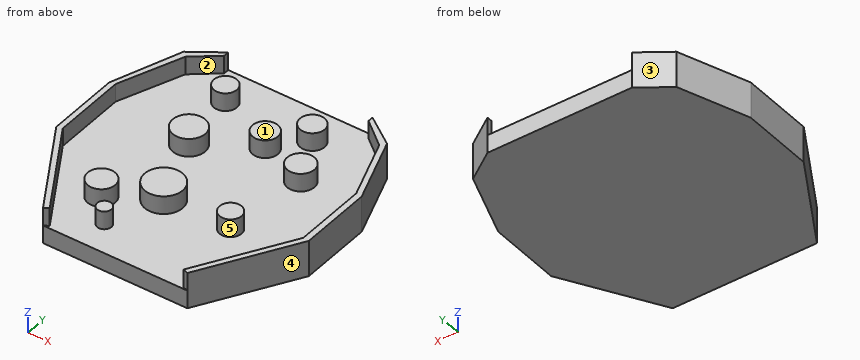
from build123d import *

# Parameters (mm, degrees)
F1_DEPTH = 2.5
F2_R     = 3.1867202998
F2_R_2   = 3.7755179731
F2_R_3   = 3.0551309049
F2_R_4   = 3.8245534148
F2_R_5   = 1.9841844708
F2_R_6   = 4.5067047705
F2_R_7   = 3.412603706
F2_R_8   = 3.5204745869
F2_R_9   = 5.26912984
F3_DEPTH = 5


with BuildPart() as f1:
    # F0 (on Top) → F1 (new body, symmetric)
    with BuildSketch(Plane.XY):
        Polygon((-28.2061724393, 29.2852179485), (0, 0), (-20, 35), align=None)
        Polygon((-20, 35), (0, 0), (20, 35), align=None)
        Polygon((20, 35), (0, 0), (28.2061724393, 29.2852179485), align=None)
        Polygon((28.2061724393, 29.2852179485), (0, 0), (35, 10.4744788063), align=None)
        Polygon((0, 0), (35, -9.5255211937), (35, 10.4744788063), align=None)
        Polygon((0, 0), (20, -35), (35, -9.5255211937), align=None)
        Polygon((-20, -35), (20, -35), (0, 0), align=None)
        Polygon((-35, -9.5255211937), (-20, -35), (0, 0), align=None)
        Polygon((-35, -9.5255211937), (0, 0), (-35, 10.4744788063), align=None)
        Polygon((-35, 10.4744788063), (0, 0), (-28.2061724393, 29.2852179485), align=None)
    extrude(amount=F1_DEPTH, both=True)

    # F2 (on face) → F3 (join)
    with BuildSketch(Plane.XY.offset(2.5)):
        with Locations((-13.5828489438, 25.1816865057)):
            Circle(F2_R)
        with Locations((16.9404093176, 12.0566859841)):
            Circle(F2_R_2)
        with Locations((14.4985457882, -11.1409882084)):
            Circle(F2_R_3)
        with Locations((-15.7194770873, -18.7718030065)):
            Circle(F2_R_4)
        with Locations((-9.3095935881, -26.402618736)):
            Circle(F2_R_5)
        with Locations((-11.1409891397, 8.0886632204)):
            Circle(F2_R_6)
        with Locations((10.5305230245, 25.1816865057)):
            Circle(F2_R_7)
        with Locations((3.5101757385, 16.940407455)):
            Circle(F2_R_8)
        with Locations((-3.8154073991, -11.4462208003)):
            Circle(F2_R_9)
        Polygon((-20, 35), (-28.2061724393, 29.2852179485), (-26.8015696019, 28.067638371), (-20, 33.5), align=None)
        Polygon((27.1522455229, 27.7875561946), (28.2061724393, 29.2852179485), (20, 35), (20, 33.5), align=None)
        Polygon((33.3497032022, 10.6280450489), (35, 10.4744788063), (28.2061724393, 29.2852179485), (27.1522455229, 27.7875561946), align=None)
        Polygon((33.3497032022, -9.3719549511), (35, -9.5255211937), (35, 10.4744788063), (33.3497032022, 10.6280450489), align=None)
        Polygon((18.5590703823, -34.4908657712), (20, -35), (35, -9.5255211937), (33.3497032022, -9.3719549511), align=None)
        Polygon((-35, -9.5255211937), (-20, -35), (-18.7074316902, -34.2389039715), (-33.5, -9.1167061117), align=None)
        Polygon((-35, 10.4744788063), (-35, -9.5255211937), (-33.5, -9.1167061117), (-33.5, 10.8832938883), align=None)
        Polygon((-28.2061724393, 29.2852179485), (-35, 10.4744788063), (-33.5, 10.8832938883), (-26.8015696019, 28.067638371), align=None)
    extrude(amount=F3_DEPTH)


solid = f1.part
Read the model definition and answer for the solid it produces. Units are mm, in the model's axes. Face numbers are marked on the shaded views. A direction names the side the tool comes from. Round coordinates to 2 decimals unless told otherwise and drop trailing zeros. Write each loop counter-clockwise with the first axis right and the second up, starting at its lowest first coordinate (ties: lowest second). Pieces come first, ordered by that corner, then holes. Notation, with made-up numbers: (23, 53) - (73, 53) arc R12 cw to (73, 75) - close; hole circle Ø6 at (-21, 24.25). An arc over 180 degrees is marked (long way). Use a Markdown table: item, result.
(1) Each of these flat-tipped pins is pushed along its axis until it touches: pin 1 Ø1.5 at (y, z) = (22, 1.5) entering from +X; pin 2 Ø1.6 at (y, z) = (34.5, 4.5) entering from +X; pin 3 Ø1.5 at (x, y) = (-20.5, 4) entering from +Z. Where does it stop, or does it pass through?
Reported:
| item | result |
|---|---|
| pin 1 | x = 31.11 |
| pin 2 | x = 21.87 |
| pin 3 | z = 2.5 |
(2) The part is cut by section D-D (x = 10). Write down the section's boundary in (y, z).
Reported:
| item | result |
|---|---|
| outline | (-35, -2.5) - (35, -2.5) - (35, 2.5) - (28.55, 2.5) - (28.55, 7.5) - (21.81, 7.5) - (21.81, 2.5) - (-35, 2.5) - close |
(3) The mould has two halves that part along Y. Classify the marked faces 1, 2 and 3: released by +Y, released by -Y, zero draft, split by the parting line, or undercut.
Reported:
| item | result |
|---|---|
| face 1 | zero draft |
| face 2 | undercut |
| face 3 | released by +Y |
(4) Straight lines are drawn through the part: line 1 along X through (y, z) = (-21, 5.75); line 2 along X through (y, z) = (20, 6.25); line 3 along Z through (x, y) = (-5.5, 15.5). For each, find the intervals that lie inside material, in ascending order. Write a range as [from, to].
Reported:
| item | result |
|---|---|
| line 1 | [-28.24, -26.5], [-18.83, -12.61], [26.5, 28.24] |
| line 2 | [-31.56, -29.95], [1.77, 5.25], [29.96, 31.56] |
| line 3 | [-2.5, 2.5] |
(5) The part is cut by section A-A (z = 4). State how many separate pieces and enclosed holes the cut face has, then the cut area to 3 significant figures.
Reported:
| item | result |
|---|---|
| separate pieces | 11 |
| enclosed holes | 0 |
| area | 628 mm2 |
(6) The part is cut by section B-B (z = 0.5). Write down the section's boundary in (x, y).
Reported:
| item | result |
|---|---|
| outline | (-35, -9.53) - (-20, -35) - (20, -35) - (35, -9.53) - (35, 10.47) - (28.21, 29.29) - (20, 35) - (-20, 35) - (-28.21, 29.29) - (-35, 10.47) - close |
(7) Which of the six approach directions +Z, -Z, +X, -X, +Y, -Y give full straight-line access (tool end or side, diameter ignored) to the marked faces 4 and 5?
Reported:
| item | result |
|---|---|
| face 4 | +Z, -Z, +X, -Y |
| face 5 | +Z |
(8) The part is cut by section C-C (y = 2.5). Write down the section's boundary in (x, z).
Reported:
| item | result |
|---|---|
| outline | (-35, -2.5) - (35, -2.5) - (35, 7.5) - (33.35, 7.5) - (33.35, 2.5) - (-33.5, 2.5) - (-33.5, 7.5) - (-35, 7.5) - close |
